Work out the finished part from the listing and answer in its coordinate system (mm). A direction names the side the tool comes from. Round coordinates to 2 decimals unless told otherwise and drop trailing zeros. Order: outer loops, then holes, each group sorted by start corner. A loop starts at its lowest first (then second) coordinate and runs counter-clockwise, first axis right, second up. Notation, with made-up numbers: M 48.5,-39.5 L 84.5,-39.5 A32 cw 84.5,-11.5 Z; hole C 1.25,78 d7. An arc over 180 degrees is marked long. Return JSON: item names as keys, results as strings.
from build123d import *

# Parameters (mm, degrees)
SKETCH1_W           = 590
SKETCH1_H           = 520
BOSS_EXTRUDE1_DEPTH = 2.7
SKETCH2_W           = 560
SKETCH2_H           = 490
BOSS_EXTRUDE2_DEPTH = 50
FILLET1_R           = 4


with BuildPart() as part:
    # Sketch1 → Boss-Extrude1 (new body)
    with BuildSketch(Plane(origin=(0, 0, 0), x_dir=(1, 0, 0), z_dir=(0, 1, 0))):
        Rectangle(SKETCH1_W, SKETCH1_H)
    extrude(amount=BOSS_EXTRUDE1_DEPTH)

    # Sketch2 → Boss-Extrude2 (add)
    with BuildSketch(Plane.XZ):
        Rectangle(SKETCH2_W, SKETCH2_H)
    extrude(amount=BOSS_EXTRUDE2_DEPTH)

    # Fillet1
    fillet1_edges = [part.edges().sort_by_distance(p)[0] for p in [
        (-295, 1.35, -260),
        (295, 1.35, -260),
        (295, 1.35, 260),
        (-295, 1.35, 260),
    ]]
    fillet(fillet1_edges, radius=FILLET1_R)


solid = part.part
Item 1: Each of these flat-tipped pins is pushed along its axis until it touches: pin 1 (1.5 mm diameter, centred on y = -41.5, z = 17.5, fed in from -X); pin 2 (5 mm diameter, centred on x = -84.5, y = -12.5, fed in from +Z); pin 3 (10 mm diameter, centred on y = -26.5, z = 135, fed in from +X). Where does it stop, or does it pass through?
Output:
{"pin 1": "stops at x = -280", "pin 2": "stops at z = 245", "pin 3": "stops at x = 280"}
Item 2: Find section A-A (x = 200.5). Determine the outline of the cut face in (y, z).
Output:
{"outline": "M -50,-245 L 0,-245 L 0,-260 L 2.7,-260 L 2.7,260 L 0,260 L 0,245 L -50,245 Z"}
Item 3: Find section C-C (y = -23.5). Determine the outline of the cut face in (x, z), plus the area to 3 significant figures.
Output:
{"outline": "M -280,-245 L 280,-245 L 280,245 L -280,245 Z", "area": "274,000 mm^2"}
Item 4: Consider line 1 along Z through (x, y) = (-247.5, -19.5); line 2 along X through (y, z) = (-22, -136). Determine where each line is inside the solid, lowest interval first. Write a range as [from, to].
Output:
{"line 1": "z = [-245, 245]", "line 2": "x = [-280, 280]"}
Item 5: Which of the six approach directions +Z, -Z, +X, -X, +Y, -Y give full straight-line access (tool end or side, diameter ignored) to faces 1 (the flat face through (280, -25, -3)), 2 (the flat face through (-4, -25, -245)), 3 (the flat face through (-280, -25, -3)), 4 (the flat face through (-4, -25, 245))?
Output:
{"face 1": "+Z, -Z, +X, -Y", "face 2": "-Z, +X, -X, -Y", "face 3": "+Z, -Z, -X, -Y", "face 4": "+Z, +X, -X, -Y"}
Item 6: Find section B-B (z = -227). Determine the outline of the cut face in (x, y).
Output:
{"outline": "M -295,0 L -280,0 L -280,-50 L 280,-50 L 280,0 L 295,0 L 295,2.7 L -295,2.7 Z"}
